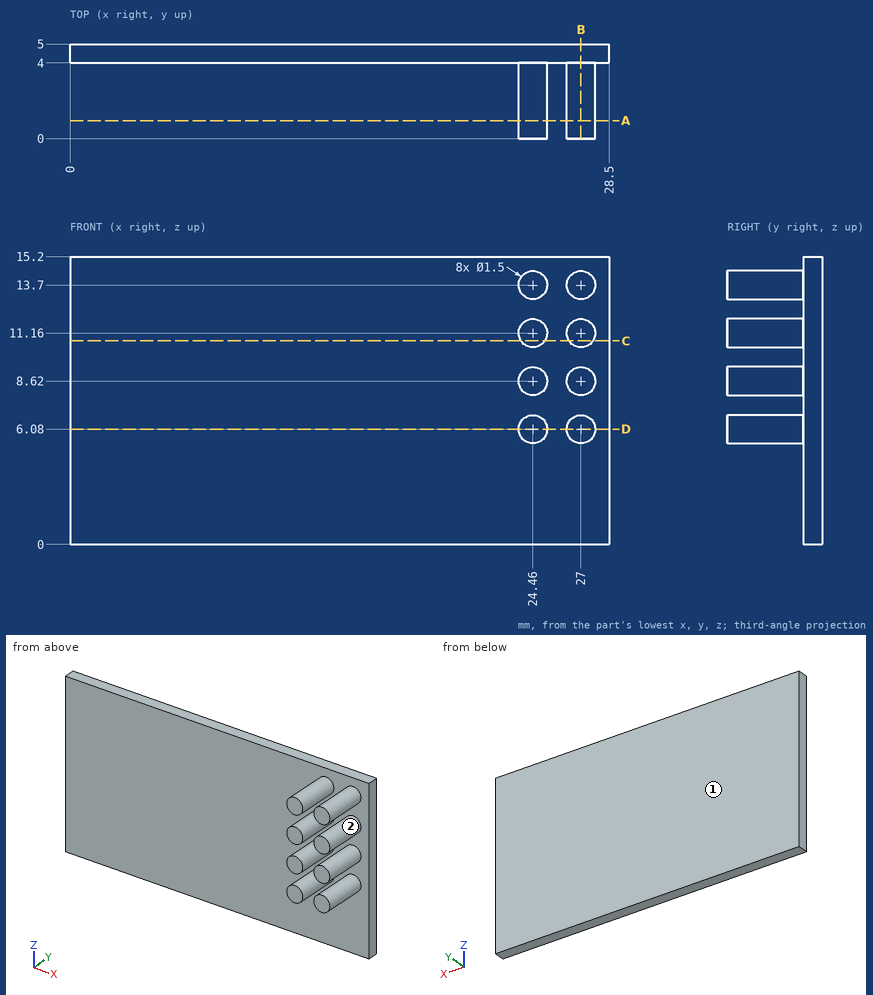
Here's the drawing with two shaded views (mm, measured from the low corner). I have some questions. Coordinates: 2 decimals unless noted, no trailing zeros. Loops run counter-clockwise (first coordinate to the right, second up) from the corner with the lowest first, then second, coordinate; pieces in that order, holes last. Notation, with made-up numbers: M -15,-25.75 L 40,-25.75 A17 ccw 40,-4.75 Z; hole C 27.25,-39 d9. An arc over 180 degrees is marked long. Put each result on its own line as item: value. Start each with the question number.
(1) We'd pull the mould along Z, two halves only. Please class the marked faces 1 and 2: +Z half, -Z half, draft (parallel to the pull), parting line (faces both ways), or undercut.
(2) I need wall thicknesses on probe 1 along X at (y, z) = (2.15, 6); probe 2 along Y at (x, z) = (2.5, 5); probe 3 along X at (y, z) = (1.6, 6.75). Which ranges of each line are inside material? Lowest first, please.
(3) Imagine slicing it at B-B on x = 27. List the corners of the cut face in (y, z) for me.
(4) Imagine slicing it at D-D on z = 6.08. List the corners of the cut face in (x, y) for me.
(5) Imagine slicing it at A-A on y = 0.95. List the corners of the cut face in (x, z) for me.
(6) Imagine slicing it at C-C on z = 10.75. List the corners of the cut face in (x, y) for me, and give its area (3 significant figures).
Worked answers:
1. face 1: draft
1. face 2: undercut
2. probe 1: x = 23.71 to 25.21, 26.25 to 27.75
2. probe 2: y = 4 to 5
2. probe 3: x = 24.12 to 24.8, 26.66 to 27.34
3. outline: M 0,5.33 L 4,5.33 L 4,0 L 5,0 L 5,15.2 L 4,15.2 L 4,14.45 L 0,14.45 L 0,12.95 L 4,12.95 L 4,11.91 L 0,11.91 L 0,10.41 L 4,10.41 L 4,9.37 L 0,9.37 L 0,7.87 L 4,7.87 L 4,6.83 L 0,6.83 Z
4. outline: M 0,4 L 23.71,4 L 23.71,0 L 25.21,0 L 25.21,4 L 26.25,4 L 26.25,0 L 27.75,0 L 27.75,4 L 28.5,4 L 28.5,5 L 0,5 Z
5. outline: C 24.46,6.08 d1.5; C 24.46,8.62 d1.5; C 24.46,11.16 d1.5; C 24.46,13.7 d1.5; C 27,6.08 d1.5; C 27,8.62 d1.5; C 27,11.16 d1.5; C 27,13.7 d1.5
6. outline: M 0,4 L 23.83,4 L 23.83,0 L 25.09,0 L 25.09,4 L 26.37,4 L 26.37,0 L 27.63,0 L 27.63,4 L 28.5,4 L 28.5,5 L 0,5 Z
6. area: 38.5 mm2
